Part model, mm, in its own coordinate system. Face numbers are marked on the shaded views. A direction names the side the tool comes from. Give positions to 0.01 mm unless a question says otherwise; leave off trailing zeros. Write each loop counter-clockwise with the first axis right and the second up, starting at its lowest first coordinate (ties: lowest second). Pieces come first, ordered by that corner, then holes. Notation, with made-up numbers: M 81,87.25 L 110,87.25 A21 ccw 110,100.25 Z; hole C 50.25,21.25 d3. An arc over 180 degrees is marked long. Use a Markdown table: item, result. Add a question column.
Autodesk Inventor part; units mm, degrees
ref_plane "YZ Plane" through (0, 0, 0) normal (1, 0, 0) x (0, 1, 0)
ref_plane "XZ Plane" through (0, 0, 0) normal (0, 1, 0) x (-1, 0, 0)
ref_plane "XY Plane" through (0, 0, 0) normal (0, 0, 1) x (1, 0, 0)
sketch "Sketch1" plane through (0, 0, 0) normal (0, 1, 0) x (-1, 0, 0)
  line L0 (0, 0) -> (-15, 0)
  line L1 (-15, 0) -> (-15, -25.825)
  line L2 (-15, -25.825) -> (0, -25.825)
  line L3 (0, -25.825) -> (0, 0)
  line L4 (-7.5, -25.825) -> (-7.5, 0) construction
  circle A0 centre (-7.5, -12.9125) radius 1.5
  line L5 (-15, -5.9125) -> (0, -5.9125)
  line L6 (0, -5.9125) -> (0, -19.9125)
  line L7 (0, -19.9125) -> (-15, -19.9125)
  line L8 (-15, -19.9125) -> (-15, -5.9125)
  line L9 (-15, -5.9125) -> (0, -19.9125) construction
  line L10 (0, -5.9125) -> (-15, -19.9125) construction
  circle A1 centre (-2.9563, -22.8688) radius 1
  circle A2 centre (-12.0437, -22.8688) radius 1
  circle A3 centre (-2.9563, -2.9563) radius 1
  circle A4 centre (-12.0438, -2.9563) radius 1
  line L11 (-5.9125, -25.825) -> (-9.0875, -25.825)
  line L12 (-9.0875, -25.825) -> (-9.0875, 0)
  line L13 (-9.0875, 0) -> (-5.9125, 0)
  line L14 (-5.9125, 0) -> (-5.9125, -25.825)
  line L15 (-5.9125, -25.825) -> (-9.0875, 0) construction
  line L16 (-9.0875, -25.825) -> (-5.9125, 0) construction
  point P0 (-15, -19.9125)
  point P1 (-15, -5.9125)
  point P2 (0, -5.9125)
  point P3 (-5.9125, -25.825)
  point P4 (-9.0875, 0)
  dimension "d0" = 15
  dimension "d2" = 3
  dimension "d3" = 12.9125
  dimension "d4" = 14
  dimension "d5" = 2
  dimension "d6" = 2.9562
  dimension "d7" = 2.9562
  dimension "d8" = 2.9562
  dimension "d9" = 2
  dimension "d11" = 2.9562
  dimension "d12" = 2.9562
  dimension "d13" = 2.9562
  dimension "d25" = 5.9125
  dimension "d68" = 3.175
  dimension "d81" = 25.825
extrude "Extrusion1" add sketch "Sketch1" against normal blind 3 contours L3 L5 L14 L0 | L14 L5 L12 L0 | L3 L7 L14 L5 | L12 L5 L1 L0 | L14 L7 L12 L5 | L3 L2 L14 L7 | L12 L7 L1 L5 | L14 L2 L12 L7 | L12 L2 L1 L7 | A0 | A1 | A2 | A3 | A4
extrude "Extrusion2" add sketch "Sketch1" against normal blind 21 contours L3 L5 L14 L0 | L14 L5 L12 L0 | L12 L5 L1 L0 | A3 | A4
hole "Hole3" at (2.9563, 0, -22.8688) at (12.0437, 0, -22.8688) direction (0, -1, 0) diameter 2.3876 end through all counterbore diameter 4.3942 counterbore depth 2
extrude "Extrusion3" cut sketch "Sketch1" against normal blind 2 contours L14 L5 L12 L0 | L14 L7 L12 L5 | L14 L2 L12 L7 | A0
sketch "Sketch3" plane through (0, -21, 0) normal (0, -1, 0) x (1, 0, 0)
  circle A0 centre (12.0437, -2.9563) radius 1
  circle A1 centre (2.9563, -2.9563) radius 1
  line L0 (15, 0) -> (0, 0)
  line L1 (15, -5.9125) -> (15, 0)
  line L2 (0, 0) -> (0, -5.9125)
  dimension "d44" = 2
  dimension "d45" = 2.9562
  dimension "d46" = 2.9562
  dimension "d47" = 2.9562
hole "Hole4" at (12.0437, -21, -2.9563) at (2.9563, -21, -2.9563) direction (0, 1, 0) diameter 1.9406 end through all
sketch "Sketch4" plane through (0, -3, 0) normal (0, -1, 0) x (1, 0, 0)
  circle A0 centre (7.5, -12.9125) radius 1.5
  point P0 (0, 0)
  dimension "d60" = 3
hole "Hole5" at (7.5, -3, -12.9125) direction (0, 1, 0) diameter 3.2004 depth 1
sketch "Sketch5" plane through (0, -21, 0) normal (0, 0, 1) x (1, 0, 0)
  circle A0 centre (7.5, 9) radius 1.5
  line L0 (0, 21) -> (5.9125, 21)
  line L1 (0, 21) -> (0, 0)
  dimension "d71" = 3
  dimension "d72" = 12
  dimension "d73" = 7.5
hole "Hole6" at (7.5, -12, 0) direction (0, 0, -1) diameter 2.459 end through all
equation "\"d3\" = 0.5 * d81"
equation "\"d6\" = d7"
equation "\"d7\" = -0.25 * d68 + 0.25 * d0"
equation "\"d8\" = d7"
equation "\"d11\" = d6"
equation "\"d12\" = d7"
equation "\"d13\" = d7"
equation "\"d25\" = 2 * d11"
equation "\"d45\" = d6"
equation "\"d46\" = d13"
equation "\"d47\" = d12"
properties part number "Bearing Sled" material "Aluminum 6061"
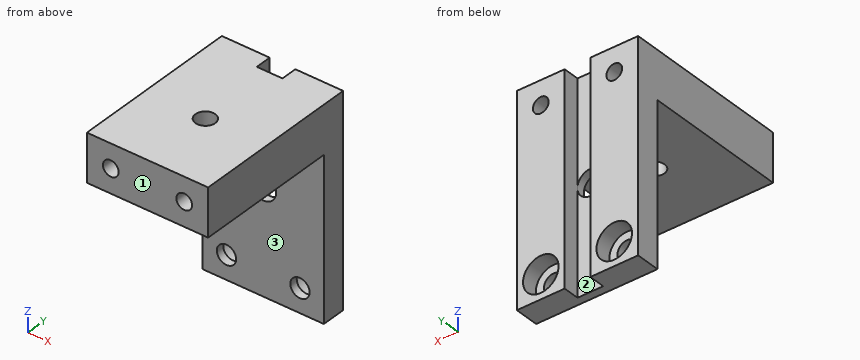
1. Drill centre lines: probe 1 along X at (y, z) = (-11.75, -3.5); probe 2 along Y at (x, z) = (4.5, -23.75); probe 3 along Z at (x, y) = (10.25, -12.5). Where is each one in solid material? Low to high. Write a range as [from, to].
2. Cut at C-C (y = -12). Write the cut outline in (x, z), then the cut area to 3 significant figures.
3. Flat gauge pins, fed straight in: pin 1 (1 mm diameter, centred on x = 7.5, z = -20, fed in from +Y); pin 2 (5 mm diameter, centred on x = 2.96, z = -22.87, fed in from -Y). Where does each tip first touch, or does it go through?
4. Cut at D-D (z = -6.5). Write the cut outline in (x, y), then the cut area to 4 significant figures.
5. Cut at B-B (z = -3.5). Write the cut outline in (x, y).
6. Tool access for the marked faces 1, 2 and 3: list every direction of +Z, -Z, +X, -X, +Y, -Y with a clear straight run to the whole face (end or side of a thin tool).
7. Cut at A-A (x = 7.5). Write the cut outline in (y, z) (1 decimal), then the cut area to 3 significant figures.
A:
| question | item | result |
|---|---|---|
| 1 | probe 1 | x = [0, 2.15], [3.76, 6.3], [8.7, 11.24], [12.85, 15] |
| 1 | probe 2 | y = [-3, -2] |
| 1 | probe 3 | z = [-5.91, 0] |
| 2 | outline | M 0,-5.91 L 6.27,-5.91 L 6.27,0 L 0,0 Z; M 8.73,-5.91 L 15,-5.91 L 15,0 L 8.73,0 Z; hole C 2.96,-2.96 d1.94; hole C 12.04,-2.96 d1.94 |
| 2 | area | 68.2 mm² |
| 3 | pin 1 | stops at y = -2 |
| 3 | pin 2 | stops at y = -3 |
| 4 | outline | M 0,-3 L 15,-3 L 15,0 L 9.09,0 L 9.09,-2 L 5.91,-2 L 5.91,0 L 0,0 Z |
| 4 | area | 38.65 mm² |
| 5 | outline | M 0,-21 L 2.15,-21 L 2.15,0 L 0,0 Z; M 3.76,-21 L 11.24,-21 L 11.24,0 L 9.09,0 L 9.09,-2 L 5.91,-2 L 5.91,0 L 3.76,0 Z; M 12.85,-21 L 15,-21 L 15,0 L 12.85,0 Z; hole C 7.5,-12 d2.46 |
| 6 | face 1 | +Z, -Z, +X, -X, -Y |
| 6 | face 2 | +Z, -Z, +Y |
| 6 | face 3 | -Z, +X, -X, -Y |
| 7 | outline | M -21,-5.9 L -13.2,-5.9 L -13.2,0 L -21,0 Z; M -10.8,-5.9 L -3,-5.9 L -3,-11.3 L -2,-11.3 L -2,0 L -10.8,0 Z; M -3,-25.8 L -2,-25.8 L -2,-14.5 L -3,-14.5 Z |
| 7 | area | 115 mm² |
